```python
from build123d import *

# Parameters (mm, degrees)
F1_DEPTH = 80


with BuildPart() as f1:
    # F0 (on Right) → F1 (new body)
    with BuildSketch(Plane.YZ):
        with BuildLine():
            Line((-25, -5), (50, -5))
            Line((50, -5), (50, 5))
            Line((50, 5), (-25, 5))
            ThreePointArc((-25, 5), (-38.462912, 7.59272), (-50, 15))
            Line((-50, 15), (-56.896552, 7.758621))
            ThreePointArc((-56.896552, 7.758621), (-42.176819, -1.692047), (-25, -5))
        make_face()
    extrude(amount=-F1_DEPTH)


solid = f1.part
```
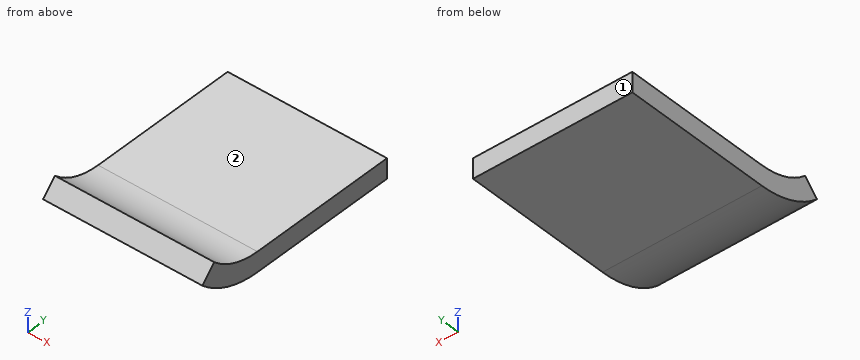
Source: CAD feature listing. Evaluate the final solid. Frame: model axes, mm. Face numbers are marked on the shaded views. A direction names the side the tool comes from. Give positions to 0.01 mm unless a question says otherwise; leave off trailing zeros. Loops run counter-clockwise (first coordinate to the right, second up) from the corner with the lowest first, then second, coordinate; pieces in that order, holes last. Notation, with made-up numbers: (7.25, -32) -> (55.25, -32) arc R13 ccw to (55.25, -18) -> close; hole circle Ø4 at (49.5, 88.25). An arc over 180 degrees is marked (long way). Use a Markdown table: item, result. Add a question column.
(1) Section query B-B (y = 24). Output: boundary loops of the cut face in (x, z).
(2) Ray query, line 1 (Z direction, x = -40.5, y = 29); line 2 (Y direction, x = -65, z = 12.25); line 3 (Y direction, x = -47, z = 13.5). Return the intervals inside material, ascending.
(3) Access query for the marked faces 1 and 2. Directions: +Z, -Z, +X, -X, +Y, -Y. A direction counts if a zero-diameter tool reaches every point of the face in a straight line with its end or side. Return the directions, or none.
(4) Section query C-C (z = -3.5). Output: boundary loops of the cut face in (x, y).
(5) First-contact query: pin 1 Ø10 at (x, y) = (-50, -26) entering from +Z; pin 2 Ø6 at (x, y) = (-43, -38.5) entering from -Z; pin 3 Ø4 at (x, z) = (-21, 12) entering from -Y. Flat tips, straight axial feed; report the tip coordinate or a pass-through.
(6) Section query A-A (x = -9). Output: boundary loops of the cut face in (y, z), then the cut area to 3 significant figures.
Checked values:
| question | item | result |
|---|---|---|
| 1 | outline | (-80, -5) -> (0, -5) -> (0, 5) -> (-80, 5) -> close |
| 2 | line 1 | -5 to 5 |
| 2 | line 2 | -52.62 to -46.75 |
| 2 | line 3 | -51.43 to -48.32 |
| 3 | face 1 | +Z, -Z, +X, -X, +Y |
| 3 | face 2 | +Z, +X, -X, +Y |
| 4 | outline | (-80, -36.68) -> (0, -36.68) -> (0, 50) -> (-80, 50) -> close |
| 5 | pin 1 | z = 5.5 |
| 5 | pin 2 | z = -3.79 |
| 5 | pin 3 | y = -54.76 |
| 6 | outline | (-56.9, 7.76) arc R46.25 ccw to (-25, -5) -> (50, -5) -> (50, 5) -> (-25, 5) arc R36.25 cw to (-50, 15) -> close |
| 6 | area | 1,060 mm^2 |
